The figure shows three views and two pictorial views of one solid part (mm, origin at its lowest corner). Answer the questions. A direction names the side the tool comes from. Give positions to 0.01 mm unless a question says otherwise; leave off trailing zeros. Write each loop counter-clockwise with the first axis right and the second up, starting at its lowest first coordinate (ties: lowest second). Pieces come first, ordered by that corner, then holes. Notation, with made-up numbers: M 30,59.25 L 56,59.25 A21 ccw 56,87.25 Z; hole C -40,67.5 d9. An arc over 180 degrees is marked long. Return JSON: item names as keys, results as strings.
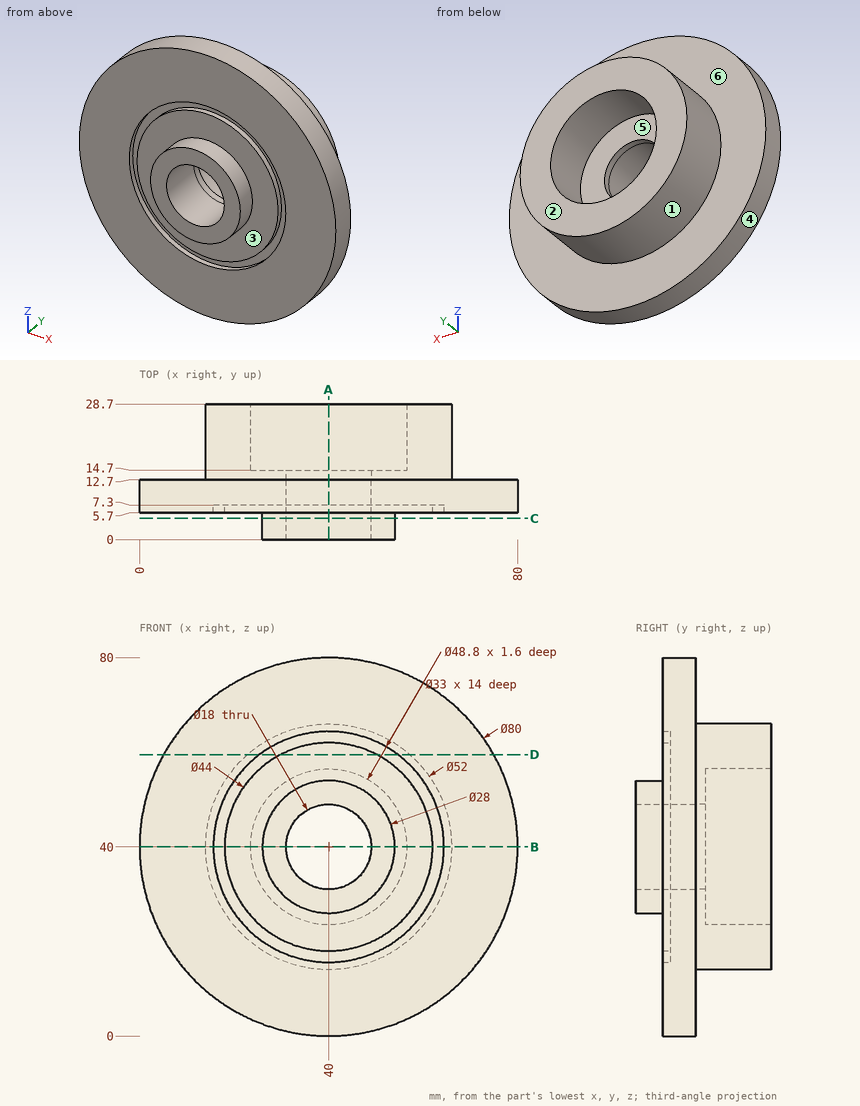
Item 1: A cutting plane is placed at C-C, the plane y = 4.5. Write down the section's boundary in (x, z).
Geometry results:
{"outline": "C 40,40 d28; hole C 40,40 d18"}
Item 2: Find the intervals of material crossed by line 1 (Z direction, x = 40, y = 17.5); line 2 (Z direction, x = 40, y = 4.75); line 3 (Y direction, x = 18, z = 57.5), in increasing order.
Geometry results:
{"line 1": "z = 14 to 23.5, 56.5 to 66", "line 2": "z = 26 to 31, 49 to 54", "line 3": "y = 5.7 to 12.7"}
Item 3: A cutting plane is placed at D-D, the plane z = 59.5. Write down the section's boundary in (x, y), plus the area to 3 significant figures.
Geometry results:
{"outline": "M 5.08,5.7 L 25.33,5.7 L 25.33,7.3 L 29.81,7.3 L 29.81,5.7 L 50.19,5.7 L 50.19,7.3 L 54.67,7.3 L 54.67,5.7 L 74.92,5.7 L 74.92,12.7 L 57.2,12.7 L 57.2,28.7 L 22.8,28.7 L 22.8,12.7 L 5.08,12.7 Z", "area": "1,020 mm2"}
Item 4: Which of the six approach directions +Z, -Z, +X, -X, +Y, -Y give full straight-line access (tool end or side, diameter ignored) to the marked faces 1, 2 and 3?
Geometry results:
{"face 1": "+Y", "face 2": "+Z, -Z, +X, -X, +Y", "face 3": "-Y"}
Item 5: Given pin 1 Ø8 at (x, y) = (71, 11) entering from +Z; pin 2 Ø8 at (x, z) = (33.5, 52) entering from -Y; pin 3 Ø6 at (y, z) = (19.5, 42.5) entering from +X; pin 4 Ø8 at (x, z) = (60, 8) entering from -Y, each flat-ended and moving along its own axis, determine where each tip first touches the part or whether it passes through.
Geometry results:
{"pin 1": "stops at z = 69.51", "pin 2": "stops at y = 0", "pin 3": "stops at x = 66", "pin 4": "stops at y = 5.7"}
Item 6: A cutting plane is placed at A-A, the plane x = 40. Write down the section's boundary in (y, z), plus the area to 3 significant figures.
Geometry results:
{"outline": "M 0,26 L 5.7,26 L 5.7,18 L 7.3,18 L 7.3,15.6 L 5.7,15.6 L 5.7,0 L 12.7,0 L 12.7,14 L 28.7,14 L 28.7,23.5 L 14.7,23.5 L 14.7,31 L 0,31 Z; M 0,49 L 14.7,49 L 14.7,56.5 L 28.7,56.5 L 28.7,66 L 12.7,66 L 12.7,80 L 5.7,80 L 5.7,64.4 L 7.3,64.4 L 7.3,62 L 5.7,62 L 5.7,54 L 0,54 Z", "area": "817 mm2"}
Item 7: Determine the mould class of the marked faces 4, 5 and 6 for opening direction X: +X half, -X half, draft (parallel to the pull), parting line (faces both ways), or undercut.
Geometry results:
{"face 4": "parting line", "face 5": "undercut", "face 6": "draft"}
Item 8: A cutting plane is placed at B-B, the plane z = 40. Write down the section's boundary in (x, y).
Geometry results:
{"outline": "M 0,5.7 L 15.6,5.7 L 15.6,7.3 L 18,7.3 L 18,5.7 L 26,5.7 L 26,0 L 31,0 L 31,14.7 L 23.5,14.7 L 23.5,28.7 L 14,28.7 L 14,12.7 L 0,12.7 Z; M 49,0 L 54,0 L 54,5.7 L 62,5.7 L 62,7.3 L 64.4,7.3 L 64.4,5.7 L 80,5.7 L 80,12.7 L 66,12.7 L 66,28.7 L 56.5,28.7 L 56.5,14.7 L 49,14.7 Z"}
